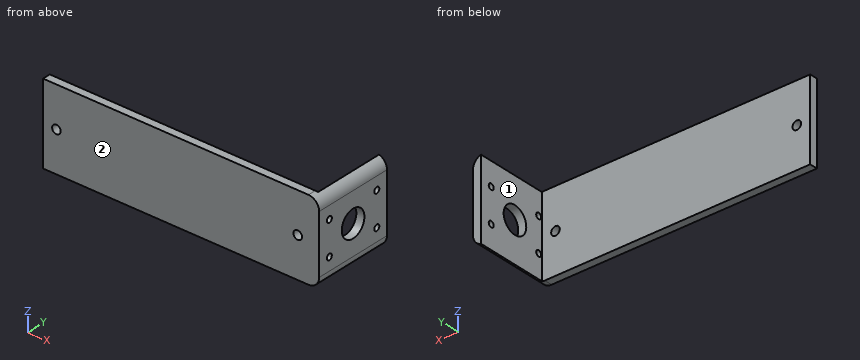
from build123d import *

# Parameters (mm, degrees)
SKETCH1_W           = 100
SKETCH1_H           = 30
BOSS_EXTRUDE1_DEPTH = 3
SKETCH2_R           = 1.6
CUT_EXTRUDE1_DEPTH  = 53.28766585
SKETCH5_W           = 30
SKETCH5_H           = 30
BOSS_EXTRUDE2_DEPTH = 3
SKETCH6_R           = 1.1
CUT_EXTRUDE2_DEPTH  = 109.323589305
SKETCH7_R           = 5
CUT_EXTRUDE3_DEPTH  = 109.323589305
FILLET1_R           = 4


with BuildPart() as part:
    # Sketch1 → Boss-Extrude1 (new body)
    with BuildSketch(Plane(origin=(0, 0, 0), x_dir=(1, 0, 0), z_dir=(0, 1, 0))):
        Rectangle(SKETCH1_W, SKETCH1_H)
    extrude(amount=BOSS_EXTRUDE1_DEPTH)

    # Sketch2 → Cut-Extrude1 (cut, through all)
    with BuildSketch(Plane(origin=(0, 3, 0), x_dir=(1, 0, 0), z_dir=(0, 1, 0))):
        with Locations(Location((45, 0, 0), (0, 0, 270))):
            Circle(SKETCH2_R)
        with Locations(Location((-45, 0, 0), (0, 0, 90))):
            Circle(SKETCH2_R)
    extrude(amount=-CUT_EXTRUDE1_DEPTH, mode=Mode.SUBTRACT)

    # Sketch5 → Boss-Extrude2 (add)
    with BuildSketch(Plane(origin=(50, 0, 0), x_dir=(0, 0, -1), z_dir=(1, 0, 0))):
        with Locations((0, 15)):
            Rectangle(SKETCH5_W, SKETCH5_H)
    extrude(amount=BOSS_EXTRUDE2_DEPTH)

    # Sketch6 → Cut-Extrude2 (cut, through all)
    with BuildSketch(Plane(origin=(53, 0, 0), x_dir=(0, 0, -1), z_dir=(1, 0, 0))):
        with Locations((-6.25, 25.5)):
            Circle(SKETCH6_R)
        with Locations(Location((6.25, 25.5, 0), (0, 0, 180))):
            Circle(SKETCH6_R)
        with Locations((6.25, 4.5)):
            Circle(SKETCH6_R)
        with Locations(Location((-6.25, 4.5, 0), (0, 0, 180))):
            Circle(SKETCH6_R)
    extrude(amount=-CUT_EXTRUDE2_DEPTH, mode=Mode.SUBTRACT)

    # Sketch7 → Cut-Extrude3 (cut, through all)
    with BuildSketch(Plane(origin=(53, 0, 0), x_dir=(0, 0, -1), z_dir=(1, 0, 0))):
        with Locations((0, 15)):
            Circle(SKETCH7_R)
    extrude(amount=-CUT_EXTRUDE3_DEPTH, mode=Mode.SUBTRACT)

    # Fillet1
    fillet1_edges = [part.edges().sort_by_distance(p)[0] for p in [
        (53, 15, -15),
        (53, 15, 15),
    ]]
    fillet(fillet1_edges, radius=FILLET1_R)


solid = part.part
Verification items for the finished model (mm, model axes). Face numbers are marked on the shaded views. A direction names the side the tool comes from. Coordinates: 2 decimals unless noted, no trailing zeros. Write each loop counter-clockwise with the first axis right and the second up, starting at its lowest first coordinate (ties: lowest second). Pieces come first, ordered by that corner, then holes. Notation, with made-up numbers: M 78.5,9 L 111.5,9 A11 cw 111.5,14 Z; hole C 85.5,28 d3. An arc over 180 degrees is marked long. One line per question, with ' | ' between items.
1) Sectioned sample at A-A on y = 25.5. Record the cut outline in (x, z).
Solutions:
outline: M 50,-14.87 A4 ccw 53,-11 L 53,-7.35 L 50,-7.35 Z; M 50,-5.15 L 53,-5.15 L 53,5.15 L 50,5.15 Z; M 50,7.35 L 53,7.35 L 53,11 A4 ccw 50,14.87 Z
2) Sectioned sample at B-B on y = 12. Record the cut outline in (x, z).
Solutions:
outline: M 50,-14.87 A4 ccw 53,-11 L 53,-4 L 50,-4 Z; M 50,4 L 53,4 L 53,11 A4 ccw 50,14.87 Z
3) Access from +Z, -Z, +X, -X, +Y, -Y to the whole of each face (thin tool, end or side, straight path). Record for the marked faces 1 and 2.
Solutions:
face 1: +Z, -Z, -X, +Y | face 2: +Z, -Z, +X, -X, -Y
4) Depth check by flat-ended pin: pin 1 Ø8 at (y, z) = (7.5, 12) entering from -X; pin 2 Ø5 at (x, z) = (-36.5, 6.5) entering from -Y; pin 3 Ø4 at (x, z) = (45, 0) entering from +Y; pin 4 Ø3 at (x, z) = (-45, 0) entering from +Y. Enter the tip coordinate at first touch or a pass-through.
Solutions:
pin 1: x = 50 | pin 2: y = 0 | pin 3: y = 3 | pin 4: through
5) Material ranges on L1, parallel to Y at x = 51.1, z = 6.25; L2, parallel to X at y = 0.65, z = 0; L3, parallel to Z at x = -45, y = 1, recorded low to high.
Solutions:
L1: 0 to 3.4, 5.6 to 24.4, 26.6 to 30 | L2: -50 to -46.6, -43.4 to 43.4, 46.6 to 53 | L3: -15 to -1.6, 1.6 to 15
6) Sectioned sample at D-D on x = -35.5. Record the cut outline in (y, z), then the cut area to 3 significant figures.
Solutions:
outline: M 0,-15 L 3,-15 L 3,15 L 0,15 Z | area: 90.0 mm^2
7) Sectioned sample at C-C on x = 45. Record the cut outline in (y, z), then the cut area to 3 significant figures.
Solutions:
outline: M 0,-15 L 3,-15 L 3,-1.6 L 0,-1.6 Z; M 0,1.6 L 3,1.6 L 3,15 L 0,15 Z | area: 80.4 mm^2
